Verification items for the finished model (mm, model axes). Face numbers are marked on the shaded views. A direction names the side the tool comes from. Give positions to 0.01 mm unless a question says otherwise; leave off trailing zeros. Loops run counter-clockwise (first coordinate to the right, second up) from the corner with the lowest first, then second, coordinate; pieces in that order, holes last. Notation, with made-up numbers: M 20,60 L 78,60 A12 ccw 78,82 Z; hole C 46.5,-26.75 d5. An arc over 180 degrees is marked long. Put each result on its own line as item: value. Start each with the question number.
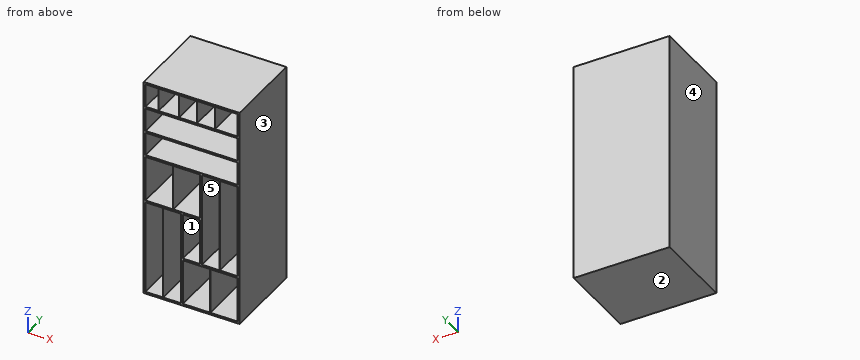
from build123d import *

# Parameters (mm, degrees)
F0_W     = 172.72
F0_H     = 19.05
F0_W_2   = 1.905
F0_H_2   = 939.8
F0_H_3   = 457.2
F0_H_4   = 234.95
F1_DEPTH = 812.8
F2_W     = 958.215
F2_H     = 2216.15
F3_DEPTH = 1.905


# Not quite as in the source:
# - a feature names something its author has since deleted; it is built from what else it names


with BuildPart() as f1:
    # F0 (on Front) → F1 (new body)
    with BuildSketch(Plane.XZ):
        Polygon((533.950886898, -1236.8191501617), (533.950886898, -1255.8691501617), (553.000886898, -1255.8691501617), (553.000886898, 960.2808498383), (533.950886898, 960.2808498383), (533.950886898, 941.2308498383), (533.950886898, 706.2808498383), (533.950886898, 687.2308498383), (533.950886898, 452.2808498383), (533.950886898, 433.2308498383), (533.950886898, 198.2808498383), (533.950886898, 179.2308498383), (533.950886898, -436.7191501617), (533.950886898, -760.5691501617), (533.950886898, -779.6191501617), align=None)
        Polygon((-212.174113102, -1236.8191501617), (-388.069113102, -1236.8191501617), (-388.069113102, -1255.8691501617), (-342.2091657827, -1255.8691501617), (532.045886898, -1255.8691501617), (533.950886898, -1255.8691501617), (533.950886898, -1236.8191501617), (532.045886898, -1236.8191501617), (260.265886898, -1236.8191501617), (258.360886898, -1236.8191501617), (-13.419113102, -1236.8191501617), (-32.469113102, -1236.8191501617), (-210.269113102, -1236.8191501617), align=None)
        Polygon((-388.069113102, -1255.8691501617), (-388.069113102, -1236.8191501617), (-388.069113102, -436.7191501617), (-388.069113102, -297.0191501617), (-388.069113102, -277.9691501617), (-388.069113102, 179.2308498383), (-388.069113102, 198.2808498383), (-388.069113102, 433.2308498383), (-388.069113102, 452.2808498383), (-386.164113102, 452.2808498383), (-386.164113102, 687.2308498383), (-386.164113102, 706.2808498383), (-386.164113102, 941.2308498383), (-259.164113102, 941.2308498383), (-257.259113102, 941.2308498383), (-54.059113102, 941.2308498383), (-52.154113102, 941.2308498383), (125.645886898, 941.2308498383), (127.550886898, 941.2308498383), (305.350886898, 941.2308498383), (307.255886898, 941.2308498383), (533.950886898, 941.2308498383), (533.950886898, 960.2808498383), (-282.659113102, 960.2808498383), (-405.214113102, 960.2808498383), (-405.214113102, -1255.8691501617), align=None)
        Polygon((-32.469113102, -297.0191501617), (-32.469113102, -1236.8191501617), (-13.419113102, -1236.8191501617), (-13.419113102, -779.6191501617), (-13.419113102, -760.5691501617), (-13.419113102, -297.0191501617), align=None)
        Polygon((-13.419113102, -760.5691501617), (-13.419113102, -779.6191501617), (258.360886898, -779.6191501617), (260.265886898, -779.6191501617), (533.950886898, -779.6191501617), (533.950886898, -760.5691501617), (356.150886898, -760.5691501617), (354.245886898, -760.5691501617), (178.350886898, -760.5691501617), (159.300886898, -760.5691501617), align=None)
        Polygon((159.300886898, -277.9691501617), (159.300886898, -297.0191501617), (159.300886898, -760.5691501617), (178.350886898, -760.5691501617), (178.350886898, 179.2308498383), (159.300886898, 179.2308498383), align=None)
        with Locations((72.940886898, -287.4941501617)):
            Rectangle(F0_W, F0_H)
        Polygon((-388.069113102, -297.0191501617), (-212.174113102, -297.0191501617), (-210.269113102, -297.0191501617), (-32.469113102, -297.0191501617), (-13.419113102, -297.0191501617), (-13.419113102, -277.9691501617), (-111.209113102, -277.9691501617), (-113.114113102, -277.9691501617), (-388.069113102, -277.9691501617), align=None)
        Polygon((-388.069113102, 198.2808498383), (-388.069113102, 179.2308498383), (-113.114113102, 179.2308498383), (-111.209113102, 179.2308498383), (159.300886898, 179.2308498383), (159.300886898, 198.2808498383), align=None)
        Polygon((533.950886898, 198.2808498383), (159.300886898, 198.2808498383), (159.300886898, 179.2308498383), (178.350886898, 179.2308498383), (354.245886898, 179.2308498383), (356.150886898, 179.2308498383), (533.950886898, 179.2308498383), align=None)
        Polygon((-388.069113102, 452.2808498383), (-388.069113102, 433.2308498383), (533.950886898, 433.2308498383), (533.950886898, 452.2808498383), (-386.164113102, 452.2808498383), align=None)
        Polygon((533.950886898, 687.2308498383), (533.950886898, 706.2808498383), (307.255886898, 706.2808498383), (305.350886898, 706.2808498383), (127.550886898, 706.2808498383), (125.645886898, 706.2808498383), (-52.154113102, 706.2808498383), (-54.059113102, 706.2808498383), (-257.259113102, 706.2808498383), (-259.164113102, 706.2808498383), (-386.164113102, 706.2808498383), (-386.164113102, 687.2308498383), align=None)
        with Locations((355.198386898, -290.6691501617)):
            Rectangle(F0_W_2, F0_H_2)
        with Locations((-112.161613102, -49.3691501617)):
            Rectangle(F0_W_2, F0_H_3)
        with Locations((-211.221613102, -766.9191501617)):
            Rectangle(F0_W_2, F0_H_2)
        with Locations((259.313386898, -1008.2191501617)):
            Rectangle(F0_W_2, F0_H_3)
        with Locations((-258.211613102, 823.7558498383)):
            Rectangle(F0_W_2, F0_H_4)
        with Locations((-53.106613102, 823.7558498383)):
            Rectangle(F0_W_2, F0_H_4)
        with Locations((126.598386898, 823.7558498383)):
            Rectangle(F0_W_2, F0_H_4)
        with Locations((306.303386898, 823.7558498383)):
            Rectangle(F0_W_2, F0_H_4)
    extrude(amount=F1_DEPTH)

    # F2 (on face) → F3 (join)
    with BuildSketch(Plane(origin=(0, 0, 0), x_dir=(-1, 0, 0), z_dir=(0, 1, 0))):
        with Locations((-73.893386898, -147.7941501617)):
            Rectangle(F2_W, F2_H)
    extrude(amount=F3_DEPTH)


solid = f1.part
Q1. Set-up check for the marked faces 4 and 5: record each of +Z, -Z, +X, -X, +Y, -Y from which the full face is reachable in a straight line by a thin tool's end or side.
Q2. Cross-section at B-B, the plane x = 444. Record the boundary of the cut face in (y, z) (3 decimals).
Q3. Scan lines: L1, parallel to X at y = -408.5, z = 113; L2, parallel to X at y = -762.5, z = -291; L3, parallel to X at y = -506, z = -851.5. Record each from-to range of solid material in increasing order.
Q4. Cross-section at D-D, the plane z = 739. Record the boundary of the cut face in (x, y) (3 decimals), then the cut area to 3 significant figures.
Q5. Release check for a two-part mould opening along Z. For the marked faces 1, 2 and 3 record: pulls with the +Z half, pulls with the -Z half, needs draft (parallel to the pull), parting line crosses it, or undercut.
Q6. Go/stop test with a flat-tipped pin: pin 1 (5 mm diameter, centred on x = -149, z = -434.5, fed in from -Y). Record where the tip stops, or that it passes through.
Q7. Cross-section at C-C, the plane y = -573. State how many separate pieces and enclosed holes the cut face has, then the cut area to 3 significant figures.
Q8. Cross-section at A-A, the plane z = 323.5. Record the boundary of the cut face in (x, y) (3 decimals), then the cut area to 3 significant figures.
Ans:
1. face 4: +Z, -Z, -X, +Y, -Y
1. face 5: -Y
2. outline: M -812.8,-1255.869 L 1.905,-1255.869 L 1.905,960.281 L -812.8,960.281 L -812.8,941.231 L 0,941.231 L 0,706.281 L -812.8,706.281 L -812.8,687.231 L 0,687.231 L 0,452.281 L -812.8,452.281 L -812.8,433.231 L 0,433.231 L 0,198.281 L -812.8,198.281 L -812.8,179.231 L 0,179.231 L 0,-760.569 L -812.8,-760.569 L -812.8,-779.619 L 0,-779.619 L 0,-1236.819 L -812.8,-1236.819 Z
3. L1: x = -405.21 to -388.07, -113.11 to -111.21, 159.3 to 178.35, 354.25 to 356.15, 533.95 to 553
3. L2: x = -405.21 to 178.35, 354.25 to 356.15, 533.95 to 553
3. L3: x = -405.21 to -388.07, -212.17 to -210.27, -32.47 to -13.42, 258.36 to 260.27, 533.95 to 553
4. outline: M -405.214,-812.8 L -386.164,-812.8 L -386.164,0 L -259.164,0 L -259.164,-812.8 L -257.259,-812.8 L -257.259,0 L -54.059,0 L -54.059,-812.8 L -52.154,-812.8 L -52.154,0 L 125.646,0 L 125.646,-812.8 L 127.551,-812.8 L 127.551,0 L 305.351,0 L 305.351,-812.8 L 307.256,-812.8 L 307.256,0 L 533.951,0 L 533.951,-812.8 L 553.001,-812.8 L 553.001,1.905 L -405.214,1.905 Z
4. area: 39,000 mm^2
5. face 1: undercut
5. face 2: pulls with the -Z half
5. face 3: needs draft
6. pin 1: stops at y = 0
7. separate pieces: 1
7. enclosed holes: 16
7. area: 233,000 mm^2
8. outline: M -405.214,-812.8 L -388.069,-812.8 L -388.069,0 L 533.951,0 L 533.951,-812.8 L 553.001,-812.8 L 553.001,1.905 L -405.214,1.905 Z
8. area: 31,200 mm^2
